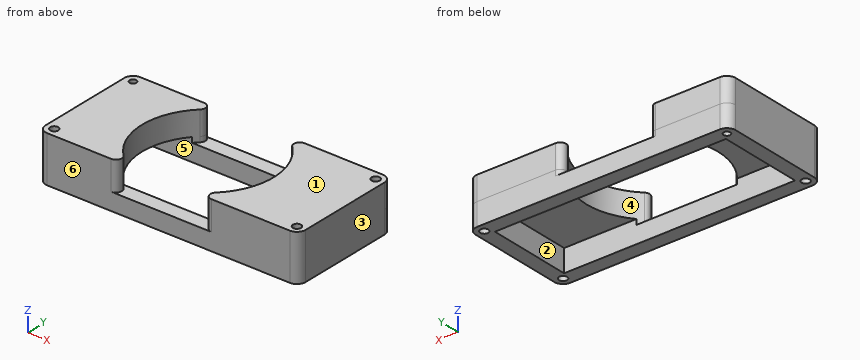
Autodesk Inventor part; units mm, degrees
ref_plane "Arbeitsebene2" through (-3.9015, -6.25, 7.6898) normal (0, 0, 1) x (1, 0, 0)
ref_plane "Arbeitsebene3" through (-21.9576, -12.7, 16.9028) normal (0, 0, -1) x (0, 1, 0)
ref_plane "YZ Plane" through (0, 0, 0) normal (1, 0, 0) x (0, 1, 0)
ref_plane "Arbeitsebene1" through (0, 0, 0) normal (0, 0, 1) x (1, 0, 0)
sketch "Skizze1" plane through (0, 0, 0) normal (0, 0, 1) x (1, 0, 0)
  circle A0 centre (57.3299, 16.4874) radius 1.4
  circle A1 centre (-25.745, -16.4874) radius 1.4
  circle A2 centre (57.3299, -16.4874) radius 1.4
  circle A3 centre (-25.745, 16.4874) radius 1.15
  circle A4 centre (9.875, 11.6896) radius 0.65
  circle A5 centre (9.875, -11.3104) radius 0.65
  circle A6 centre (14.955, 11.6896) radius 0.65
  circle A7 centre (14.955, -11.3104) radius 0.65
  circle A8 centre (25.115, 11.6896) radius 0.65
  circle A9 centre (25.115, -11.3104) radius 0.65
  circle A10 centre (30.195, 11.6896) radius 0.65
  circle A11 centre (30.195, -11.3104) radius 0.65
  circle A12 centre (-2.825, -11.3104) radius 0.65
  circle A13 centre (-2.825, 11.6896) radius 0.65
  circle A14 centre (-0.285, -11.3104) radius 0.65
  circle A15 centre (-0.285, 11.6896) radius 0.65
  circle A16 centre (2.255, -11.3104) radius 0.65
  circle A17 centre (2.255, 11.6896) radius 0.65
  circle A18 centre (4.795, -11.3104) radius 0.65
  circle A19 centre (4.795, 11.6896) radius 0.65
  circle A20 centre (27.655, -11.3104) radius 0.65
  circle A21 centre (27.655, 11.6896) radius 0.65
  circle A22 centre (22.575, -11.3104) radius 0.65
  circle A23 centre (22.575, 11.6896) radius 0.65
  circle A24 centre (17.495, -11.3104) radius 0.65
  circle A25 centre (17.495, 11.6896) radius 0.65
  circle A26 centre (12.415, -11.3104) radius 0.65
  circle A27 centre (12.415, 11.6896) radius 0.65
  circle A28 centre (7.335, -11.3104) radius 0.65
  circle A29 centre (7.335, 11.6896) radius 0.65
  circle A30 centre (20.035, 11.6896) radius 0.65
  circle A31 centre (20.035, -11.3104) radius 0.65
  arc A32 (-28.745, -16.4874) -> (-25.745, -19.4874) centre (-25.745, -16.4874) ccw
  line L0 (57.3299, -19.4874) -> (-25.745, -19.4874)
  arc A33 (57.3299, -19.4874) -> (60.3299, -16.4874) centre (57.3299, -16.4874) ccw
  line L1 (60.3299, 16.4874) -> (60.3299, -16.4874)
  arc A34 (60.3299, 16.4874) -> (57.3299, 19.4874) centre (57.3299, 16.4874) ccw
  line L2 (-25.745, 19.4874) -> (57.3299, 19.4874)
  arc A35 (-25.745, 19.4874) -> (-28.745, 16.4874) centre (-25.745, 16.4874) ccw
  line L3 (-28.745, -16.4874) -> (-28.745, 16.4874)
  line L4 (55.3299, 14.4874) -> (55.3299, -14.4874)
  line L5 (55.3299, -14.4874) -> (-23.745, -14.4874)
  line L6 (-23.745, -14.4874) -> (-23.745, 14.4874)
  line L7 (-23.745, 14.4874) -> (55.3299, 14.4874)
  point P0 (0, 0)
  dimension "d0" = 5
ref_plane "Arbeitsebene2" through (-3.9015, -6.25, 7.6898) normal (0, 0, 1) x (1, 0, 0)
extrude "Extrusion1" add sketch "Skizze1" along normal up to surface (7.6898 mm away) contours L3 A35 L2 A34 L1 A33 L0 A32
sketch "Skizze2" plane through (-25.745, -19.4874, 7.6898) normal (0, 0, 1) x (1, 0, 0)
  circle A0 centre (83.0749, 35.9749) radius 1.4
  circle A1 centre (0, 3) radius 1.4
  circle A2 centre (83.0749, 3) radius 1.4
  circle A3 centre (0, 35.9749) radius 1.15
  line L0 (81.0749, 33.9749) -> (2, 33.9749)
  line L1 (81.0749, 5) -> (81.0749, 33.9749)
  line L2 (2, 5) -> (81.0749, 5)
  line L3 (2, 33.9749) -> (2, 5)
  arc A4 (0, 38.9749) -> (-3, 35.9749) centre (0, 35.9749) ccw
  line L4 (-3, 3) -> (-3, 35.9749)
  arc A5 (-3, 3) -> (0, 0) centre (0, 3) ccw
  line L5 (83.0749, 0) -> (0, 0)
  arc A6 (83.0749, 0) -> (86.0749, 3) centre (83.0749, 3) ccw
  line L6 (86.0749, 35.9749) -> (86.0749, 3)
  arc A7 (86.0749, 35.9749) -> (83.0749, 38.9749) centre (83.0749, 35.9749) ccw
  line L7 (0, 38.9749) -> (83.0749, 38.9749)
  circle A8 centre (39.0935, 19.4874) radius 3.8655
  line L8 (43.0093, 18.0044) -> (43.0093, 15.5716)
  line L9 (43.0093, 15.322) -> (35.1777, 15.322)
  line L10 (35.1777, 23.4033) -> (37.6105, 23.4033)
  line L11 (34.9281, 15.5716) -> (34.9281, 23.4033)
  line L12 (43.3435, 23.4874) -> (43.3435, 15.4874)
  line L13 (35.0935, 23.7374) -> (43.0935, 23.7374)
  line L14 (34.9281, 15.5716) -> (34.9281, 23.4033)
  line L15 (34.9935, 15.3874) -> (43.1935, 15.3874)
  line L16 (43.1935, 15.3874) -> (43.1935, 23.5874)
  line L17 (43.1935, 23.5874) -> (34.9935, 23.5874)
  line L18 (34.9935, 23.5874) -> (34.9935, 15.3874)
  line L19 (34.9935, 15.3874) -> (43.1935, 23.5874) construction
  line L20 (43.1935, 15.3874) -> (34.9935, 23.5874) construction
  point P0 (25.745, 19.4874)
  dimension "d3" = 8.2
  dimension "d4" = 8.2
extrude "Extrusion2" add sketch "Skizze2" along normal blind 2.2 contours L1 L2 L3 L0 | L7 A7 L6 A6 L5 A5 L4 A4
ref_plane "Arbeitsebene3" through (-21.9576, -12.7, 16.9028) normal (0, 0, -1) x (0, 1, 0)
sketch "Skizze3" plane through (-25.745, -19.4874, 9.8898) normal (0, 0, 1) x (1, 0, 0)
  line L0 (83.0749, 38.9749) -> (0, 38.9749)
  arc A0 (0, 38.9749) -> (-3, 35.9749) centre (0, 35.9749) ccw
  line L1 (-3, 35.9749) -> (-3, 3)
  arc A1 (-3, 3) -> (0, 0) centre (0, 3) ccw
  line L2 (0, 0) -> (83.0749, 0)
  arc A2 (83.0749, 0) -> (86.0749, 3) centre (83.0749, 3) ccw
  line L3 (86.0749, 3) -> (86.0749, 35.9749)
  arc A3 (86.0749, 35.9749) -> (83.0749, 38.9749) centre (83.0749, 35.9749) ccw
  line L4 (34.9935, 15.3874) -> (34.9935, 23.5874)
  line L5 (34.9935, 23.5874) -> (43.1935, 23.5874)
  line L6 (43.1935, 23.5874) -> (43.1935, 15.3874)
  line L7 (43.1935, 15.3874) -> (34.9935, 15.3874)
  circle A4 centre (0, 35.9749) radius 1.15
  circle A5 centre (83.0749, 3) radius 1.4
  circle A6 centre (0, 3) radius 1.4
  circle A7 centre (83.0749, 35.9749) radius 1.4
  circle A8 centre (39.0935, 19.4874) radius 3.6158
  circle A9 centre (39.0935, 19.4874) radius 3.475
  point P0 (25.745, 19.4874)
  dimension "d7" = 6.95
extrude "Extrusion3" add sketch "Skizze3" along normal blind 6 contours A3 L3 A2 L2 A1 L1 A0 L0 | L4 L5 L6 L7
sketch "Skizze4" plane through (-25.745, 19.4874, 15.8898) normal (0, 0, 1) x (1, 0, 0)
  circle A0 centre (39.0935, -19.4874) radius 3.6158
  circle A1 centre (39.0935, -19.4874) radius 22.5
  point P0 (25.745, -19.4874)
  dimension "d10" = 45
extrude "Extrusion4" cut sketch "Skizze4" against normal blind 10
ref_plane "Arbeitsebene4" through (-25.745, 0, 0) normal (0, -1, 0) x (1, 0, 0)
fillet "Rundung1" radius 2 4 edges at (2.1017, -19.4874, 10.8898) (24.5952, -19.4874, 10.8898) (2.1017, 19.4874, 10.8898) (24.5952, 19.4874, 10.8898)
thread "Gewinde1"
properties part number "ESP32ParasiteMicroscope_middle_v0"
Can you work these out from the model? Positions are in its coordinate system, mm. Face numbers are marked on the shaded views. A direction names the side the tool comes from. Give positions to 0.01 mm unless a question says otherwise; leave off trailing zeros. Loops run counter-clockwise (first coordinate to the right, second up) from the corner with the lowest first, then second, coordinate; pieces in that order, holes last. Notation, with made-up numbers: M 8,68.5 L 48,68.5 A18 ccw 48,98.5 Z; hole C 88,28.5 d8. An arc over 180 degrees is marked long. Answer in a Markdown table with one row per item.
1. If I drill on line 1 along X through (y, z) = (1.5, 3.75) (3 decimals); line 2 along Y through (x, z) = (-12.5, 5.25); line 3 along Z through (x, y) = (-7.5, 12.5), over which ranges is the centre line in solid material (lowest first)?
Taken from the geometry:
| item | result |
|---|---|
| line 1 | x = -28.745 to -23.745, 55.33 to 60.33 |
| line 2 | y = -19.49 to -14.49, 14.49 to 19.49 |
| line 3 | z = 7.69 to 15.89 |
2. For pin 1 Ø5.5 at (x, y) = (6, 17) entering from +Z; pin 2 Ø2 at (x, y) = (-25.74, 16.49) entering from -Z; pin 3 Ø1.5 at (x, y) = (50.5, 7.5) entering from -Z, each with a flat end and sliding along its axis, tell me the tip position at first contact or that it passes through.
Taken from the geometry:
| item | result |
|---|---|
| pin 1 | stops at z = 5.89 |
| pin 2 | passes through |
| pin 3 | stops at z = 7.69 |
3. Suppose I cut it at C-C on y = 0.5. Write out the boundary of the cut face in (x, z) (3 decimals), plus the area to 3 significant figures.
Taken from the geometry:
| item | result |
|---|---|
| outline | M -28.745,0 L -23.745,0 L -23.745,7.69 L -9.146,7.69 L -9.146,15.89 L -28.745,15.89 Z; M 35.843,7.69 L 55.33,7.69 L 55.33,0 L 60.33,0 L 60.33,15.89 L 35.843,15.89 Z |
| area | 438 mm² |
4. Suppose I cut it at B-B on z = 5. Write out the boundary of the cut face in (x, y) (3 decimals), plus the area to 3 significant figures.
Taken from the geometry:
| item | result |
|---|---|
| outline | M -28.745,-16.487 A3 ccw -25.745,-19.487 L 57.33,-19.487 A3 ccw 60.33,-16.487 L 60.33,16.487 A3 ccw 57.33,19.487 L -25.745,19.487 A3 ccw -28.745,16.487 Z; hole C -25.745,-16.487 d2.8; hole C -25.745,16.487 d2.3; hole M -23.745,-14.487 L 55.33,-14.487 L 55.33,14.487 L -23.745,14.487 Z; hole C 57.33,-16.487 d2.8; hole C 57.33,16.487 d2.8 |
| area | 1,150 mm² |
5. Thinking about a two-plate mould opening in X: for the marked faces 1, 2 and 3, which applies, released by +X, released by -X, zero draft, split by the parting line, or undercut?
Taken from the geometry:
| item | result |
|---|---|
| face 1 | zero draft |
| face 2 | undercut |
| face 3 | released by +X |
6. Suppose I cut it at D-D on x = -21. Write out the boundary of the cut face in (y, z), plus the area to 3 significant figures.
Taken from the geometry:
| item | result |
|---|---|
| outline | M -19.49,0 L -14.49,0 L -14.49,7.69 L 14.49,7.69 L 14.49,0 L 19.49,0 L 19.49,15.89 L -19.49,15.89 Z |
| area | 396 mm² |
7. Suppose I cut it at A-A on x = 15. Write out the boundary of the cut face in (y, z), plus the area to 3 significant figures.
Taken from the geometry:
| item | result |
|---|---|
| outline | M -19.49,0 L -14.49,0 L -14.49,5.89 L -19.49,5.89 Z; M 14.49,0 L 19.49,0 L 19.49,5.89 L 14.49,5.89 Z |
| area | 58.9 mm² |
8. Which directions (+Z, -Z, +X, -X, +Y, -Y) give clear straight access to the entire face, cutting with the end or side of a thin tool? Please do the marked faces 4, 5 and 6.
Taken from the geometry:
| item | result |
|---|---|
| face 4 | +Z |
| face 5 | -Z |
| face 6 | +Z, -Z, +X, -X, -Y |
